from build123d import *

# Parameters (mm, degrees)
F0_R     = 11
F1_DEPTH = 3
F2_R     = 10
F3_DEPTH = 2


with BuildPart() as f1:
    # F0 (on Top) → F1 (new body)
    with BuildSketch(Plane.XY):
        Circle(F0_R)
    extrude(amount=F1_DEPTH)

    # F2 (on face) → F3 (cut)
    with BuildSketch(Plane.XY.offset(3)):
        Circle(F2_R)
    extrude(amount=-F3_DEPTH, mode=Mode.SUBTRACT)

    # F4 (on Front) → F5 (revolve)
    with BuildSketch(Plane.XZ):
        with BuildLine():
            add(Edge.make_bspline(
                [(-10, 3), (-9.5631365163, 3.1947120998), (-8.9358639257, 3.1521992443), (-8.3988746628, 3)],
                knots=[0, 0, 0, 0, 0.1598537325, 0.1598537325, 0.1598537325, 0.1598537325], degree=3))
            Line((-10, 3), (-8.3988746628, 3))
        make_face()
        with BuildLine():
            Line((-8.3988746628, 3), (-10, 3))
            Line((-10, 3), (-10, 2.2))
            Line((-10, 2.2), (0, 2.2))
            Line((0, 2.2), (0, 3))
            Line((0, 3), (-2.2816949674, 3))
            add(Edge.make_bspline(
                [(-4.2584559222, 3), (-3.9238062504, 2.8445189646), (-3.2540976505, 2.5415343681), (-2.5906789659, 2.8182773792), (-2.2816949674, 3)],
                knots=[0.5757910273, 0.5757910273, 0.5757910273, 0.5757910273, 0.6661755998, 0.754812685, 0.754812685, 0.754812685, 0.754812685], degree=3))
            Line((-4.2584559222, 3), (-6.2872854841, 3))
            add(Edge.make_bspline(
                [(-8.3988746628, 3), (-7.8910468525, 2.8560660067), (-7.2552687251, 2.4957672366), (-6.5324171697, 2.8740056535), (-6.2872854841, 3)],
                knots=[0.1598537325, 0.1598537325, 0.1598537325, 0.1598537325, 0.3110265335, 0.3848969639, 0.3848969639, 0.3848969639, 0.3848969639], degree=3))
        make_face()
        with BuildLine():
            add(Edge.make_bspline(
                [(-6.2872854841, 3), (-5.9671465556, 3.1645470474), (-5.3071713867, 3.4963401186), (-4.6080475442, 3.1624231904), (-4.2584559222, 3)],
                knots=[0.3848969639, 0.3848969639, 0.3848969639, 0.3848969639, 0.4813708261, 0.5757910273, 0.5757910273, 0.5757910273, 0.5757910273], degree=3))
            Line((-6.2872854841, 3), (-4.2584559222, 3))
        make_face()
        with BuildLine():
            Line((-2.2816949674, 3), (0, 3))
            Line((0, 3), (0, 4))
            add(Edge.make_bspline(
                [(-2.2816949674, 3), (-1.9564930944, 3.191260832), (-1.1585189995, 3.8240848781), (-0.654182455, 4.0144366212), (0, 4)],
                knots=[0.754812685, 0.754812685, 0.754812685, 0.754812685, 0.8481021313, 1, 1, 1, 1], degree=3))
        make_face()
    revolve(axis=Axis((0, 0, 3.1), (0, 0, 1)))


solid = f1.part
Could you check a few things on this model? Use its own coordinates, in mm. A direction names the side the tool comes from. Give positions to 0.01 mm unless a question says otherwise; leave off trailing zeros. Loops run counter-clockwise (first coordinate to the right, second up) from the corner with the lowest first, then second, coordinate; pieces in that order, holes last. Notation, with made-up numbers: (40, -32.5) -> (52, -32.5) arc R11 ccw to (52, -28.5) -> close; hole circle Ø2 at (1.25, 73). An arc over 180 degrees is marked (long way). Answer as CSV lines item,"result". Start each with the question number.
(1) I'm going to push a flat-ended pin straight in: pin 1 Ø10 at (x, y) = (5, -7) entering from +Z. Where does the tip first touch, or does it pass through?
(2) Which directions (+Z, -Z, +X, -X, +Y, -Y) give clear straight access to the entire face, cutting with the end or side of a thin tool? Please do faces 1 (the flat face through (0, 0, 0)), 2 (the flat face through (0, 0, 1)).
(3) If we section it at A-A on z = 1.65: Write out the boundary of the cut face in (x, y).
(4) I need wall thicknesses on probe 1 along Z at (x, y) = (-4.75, -5.25); probe 2 along Y at (x, z) = (0, 1.75); probe 3 along Z at (x, y) = (-1.5, -1.75). Which ranges of each line are inside material? Lowest first, please.
(5) We'd pull the mould along X, two halves only. Please class faces 3 (the cylindrical face through (-2.38, -10.74, 1.48)), 4 (the flat face through (2, -10, 3)), 5 (the flat face through (0, 0, 2.2)): released by +X, released by -X, zero draft, split by the parting line, or undercut.
Computed:
1,pin 1,"stops at z = 3.33"
2,face 1,"-Z, +X, -X, +Y, -Y"
2,face 2,"none"
3,outline,"circle Ø22 at (0, 0); hole circle Ø20 at (0, 0)"
4,probe 1,"z = 0 to 1, 2.2 to 2.69"
4,probe 2,"y = -11 to -10, 10 to 11"
4,probe 3,"z = 0 to 1, 2.2 to 2.99"
5,face 3,"split by the parting line"
5,face 4,"zero draft"
5,face 5,"undercut"
